```python
from build123d import *

# Parameters (mm, degrees)
F0_W           = 20
F0_H           = 20
F1_DEPTH       = 30
F2_SIZE        = 17.5
F4_D           = 5
F4_CSINK_D     = 9
F4_CSINK_ANGLE = 90


with BuildPart() as f1:
    # F0 (on Top) → F1 (new body)
    with BuildSketch(Plane.XY):
        with Locations((-4.093967, -2.481039)):
            Rectangle(F0_W, F0_H)
    extrude(amount=F1_DEPTH)

    # F2
    f2_edges = [f1.edges().sort_by_distance(p)[0] for p in [
        (-4.093967, -12.481039, 30),
    ]]
    chamfer(f2_edges, length=F2_SIZE)

    # F4 (through all)
    with Locations(Plane(origin=(0, 0, 0), x_dir=(1, 0, 0), z_dir=(0, 0, -1))):
        with Locations((-4.093967, 6.481039)):
            CounterSinkHole(F4_D / 2, F4_CSINK_D / 2, counter_sink_angle=F4_CSINK_ANGLE)


solid = f1.part
```
Could you check a few things on this model? Use its own coordinates, in mm. Give positions to 0.01 mm unless a question says otherwise; leave off trailing zeros. Order: outer loops, then holes, each group sorted by start corner. A loop starts at its lowest first (then second) coordinate and runs counter-clockwise, first axis right, second up.
Q1. Suppose I cut it at A-A, the plane x = 1. Write out the boundary of the cut face in (y, z).
Q2. We'd pull the mould along X, two halves only. Please class faces 1 (the cylindrical face through (-3.55, -4.04, 9.52)), 2 (the flat face through (-4.23, -3.61, 21.37)), 3 (the flat face through (5.906, 0, 11)): +X half, -X half, draft (parallel to the pull), parting line (faces both ways), or undercut.
Q3. Suppose I cut it at D-D, the plane z = 19.75. Write out the boundary of the cut face in (x, y).
Q4. I'm going to push flat-ended pins straight in: P1, Ø3, axis at x = -4.09, y = -6.48, coming from the +Z side; P2, Ø10, axis at x = -4, y = -5, coming from the +Z side. Where does each tip first touch, or does it pass through?
Q5. If I drill on line 1 along Y through (x, z) = (-5.75, 21); line 2 along Y through (x, z) = (-2.75, 13.75); line 3 along X through (y, z) = (-4.25, 17.75), over which ranges is the centre line in solid material (lowest first)?
Q6. Suppose I cut it at C-C, the plane y = 3. Write out the boundary of the cut face in (x, z).
Q7. Suppose I cut it at B-B, the plane z = 11. Write out the boundary of the cut face in (x, y).
Solution:
1. outline: (-12.48, 0) - (7.52, 0) - (7.52, 30) - (5.02, 30) - (-12.48, 12.5) - close
2. face 1: undercut
2. face 2: draft
2. face 3: +X half
3. outline: (-14.09, -5.23) - (-6.26, -5.23) arc R2.5 cw to (-1.93, -5.23) - (5.91, -5.23) - (5.91, 7.52) - (-14.09, 7.52) - close
4. P1: passes through
4. P2: stops at z = 24.98
5. line 1: y = -3.98 to 7.52
5. line 2: y = -11.23 to -8.59, -4.37 to 7.52
5. line 3: x = -14.09 to -5.22, -2.97 to 5.91
6. outline: (-14.09, 0) - (5.91, 0) - (5.91, 27.98) - (-14.09, 27.98) - close
7. outline: (-14.09, -12.48) - (5.91, -12.48) - (5.91, 7.52) - (-14.09, 7.52) - close; hole circle Ø5 at (-4.09, -6.48)
